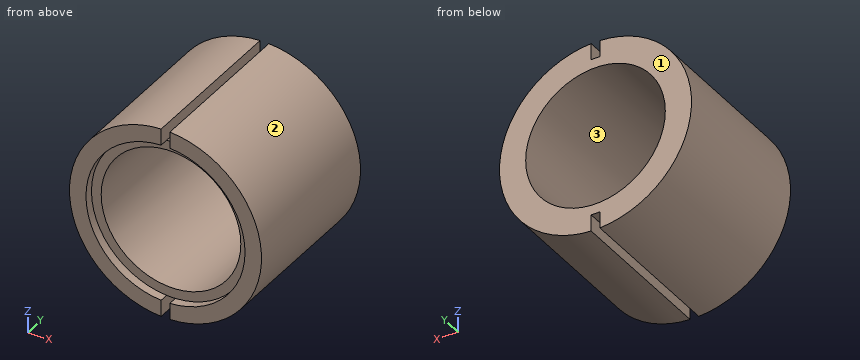
```python
from build123d import *

# Parameters (mm, degrees)
F0_R     = 11
F0_R_2   = 9.1123830153
F1_DEPTH = 18
F3_DEPTH = 25
F0_R_3   = 8
F4_DEPTH = 17


with BuildPart() as f1:
    # F0 (on Front) → F1 (new body)
    with BuildSketch(Plane.XZ):
        Circle(F0_R)
        Circle(F0_R_2, mode=Mode.SUBTRACT)
    extrude(amount=F1_DEPTH)

    # F2 (on Front) → F3 (cut)
    with BuildSketch(Plane.XZ):
        Polygon((-0.5, 11.3087910658), (-0.5, 1.3087910658), (0.5, 1.3087910658), (0.5, 11.2789400049), align=None)
        Polygon((0.5, -1.3087910658), (-0.5, -1.3087910658), (-0.5, -11.3087910658), (0.5, -11.2789400049), align=None)
    extrude(amount=F3_DEPTH, mode=Mode.SUBTRACT)

    # F0 (on Front) → F4 (join)
    with BuildSketch(Plane.XZ):
        Circle(F0_R_2)
        Circle(F0_R_3, mode=Mode.SUBTRACT)
    extrude(amount=F4_DEPTH)


solid = f1.part
```
Check sheet for the modelled part. Datum: model origin and axes. Units: mm. Face numbers are marked on the shaded views. Round coordinates to 2 decimals unless told otherwise and drop trailing zeros. Order: outer loops, then holes, each group sorted by start corner. A loop starts at its lowest first (then second) coordinate and runs counter-clockwise, first axis right, second up. Notation, with made-up numbers: M 52,-36 L 73,-36 A30 cw 73,-1 Z; hole C 89,76.5 d5. An arc over 180 degrees is marked long. Answer in a Markdown table with one row per item.
(1) Section check D-D on z = -3.5. Record the boundary of the cut face in (x, y), plus the area to 3 significant figures.
Findings:
| item | result |
|---|---|
| outline | M -10.43,-18 L -8.41,-18 L -8.41,-17 L -7.19,-17 L -7.19,0 L -10.43,0 Z; M 7.19,-17 L 8.41,-17 L 8.41,-18 L 10.43,-18 L 10.43,0 L 7.19,0 Z |
| area | 114 mm^2 |
(2) Draft check along X on the marked faces 1, 2 and 3. Enter one of: +X half, -X half, draft (parallel to the pull), parting line (faces both ways), or undercut.
Findings:
| item | result |
|---|---|
| face 1 | draft |
| face 2 | +X half |
| face 3 | undercut |
(3) Section check C-C on z = 0. Record the boundary of the cut face in (x, y).
Findings:
| item | result |
|---|---|
| outline | M -11,-18 L -9.11,-18 L -9.11,-17 L -8,-17 L -8,0 L -11,0 Z; M 8,-17 L 9.11,-17 L 9.11,-18 L 11,-18 L 11,0 L 8,0 Z |
(4) Gauge pin test, flat ends, axial feed: pin 1 (1 mm diameter, centred on x = 3, y = -5.5, fed in from -Z); pin 2 (6 mm diameter, centred on y = -7, z = 8, fed in from +X); pin 3 (4 mm diameter, centred on y = -5.5, z = 8, fed in from -X); pin 4 (3 mm diameter, centred on x = 7.5, z = 4, fed in from -Y). Record the tip position at first contact, or that the pin passes through.
Findings:
| item | result |
|---|---|
| pin 1 | stops at z = -10.71 |
| pin 2 | stops at x = 9.8 |
| pin 3 | stops at x = -9.22 |
| pin 4 | stops at y = -18 |
(5) Section check B-B on x = 0. Record the boundary of the cut face in (y, z).
Findings:
| item | result |
|---|---|
| outline | M -17,-9.11 L 0,-9.11 L 0,-8 L -17,-8 Z; M -17,8 L 0,8 L 0,9.11 L -17,9.11 Z |
(6) Material ranges on line 1 along Z through (x, y) = (0, -8.5); line 2 along Y through (x, z) = (-1.25, -8); line 3 along Z through (x, y) = (6.75, -15.75), recorded low to high. Write a range as from..to.
Findings:
| item | result |
|---|---|
| line 1 | z = -9.11..-8, 8..9.11 |
| line 2 | y = -17..0 |
| line 3 | z = -8.69..-4.29, 4.29..8.69 |
(7) Section check A-A on y = -16.25. Record the boundary of the cut face in (x, z).
Findings:
| item | result |
|---|---|
| outline | M -0.5,-10.99 L -0.5,-9.1 A9.11 ccw 0.5,-9.1 L 0.5,-10.99 A11 ccw 0.5,10.99 L 0.5,9.1 A9.11 ccw -0.5,9.1 L -0.5,10.99 A11 ccw Z; hole C 0,0 d16 |
